```python
from build123d import *

# Parameters (mm, degrees)
F0_W     = 521
F0_H     = 278
F0_W_2   = 117
F0_H_2   = 168
F1_DEPTH = 2


with BuildPart() as f1:
    # F0 (on Front) → F1 (new body)
    with BuildSketch(Plane.XZ):
        Rectangle(F0_W, F0_H)
        with Locations((-147, 0)):
            Rectangle(F0_W_2, F0_H_2, mode=Mode.SUBTRACT)
        Rectangle(F0_W_2, F0_H_2, mode=Mode.SUBTRACT)
        with Locations((147, 0)):
            Rectangle(F0_W_2, F0_H_2, mode=Mode.SUBTRACT)
    extrude(amount=F1_DEPTH)


solid = f1.part
```
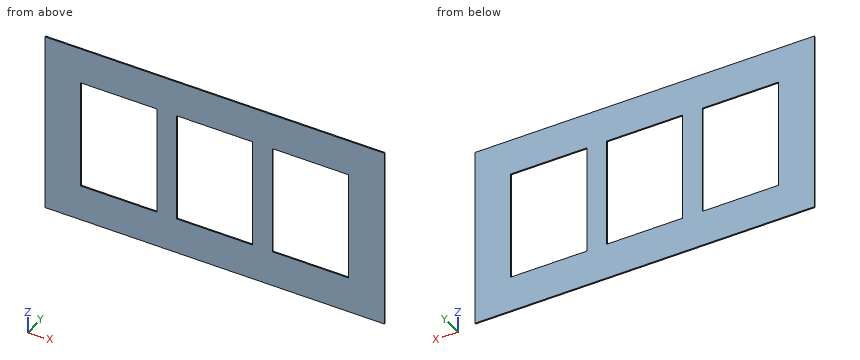
The model under review builds one solid part; all positions refer to its coordinate system, in mm. Round coordinates to 2 decimals unless told otherwise and drop trailing zeros. Order: outer loops, then holes, each group sorted by start corner. A loop starts at its lowest first (then second) coordinate and runs counter-clockwise, first axis right, second up.
Item 1: To check wall thickness, follow probe 1 along X at (y, z) = (-0.2, 8); probe 2 along Z at (x, y) = (168.5, -1.75). State the ranges of each line that lie inside material, in increasing order.
Working result:
probe 1: x = -260.5 to -205.5, -88.5 to -58.5, 58.5 to 88.5, 205.5 to 260.5
probe 2: z = -139 to -84, 84 to 139
Item 2: Add section C-C, the plane y = -0.95. State the section outline as (x, z) points, and give its area (3 significant figures).
Working result:
outline: (-260.5, -139) - (260.5, -139) - (260.5, 139) - (-260.5, 139) - close; hole (-205.5, -84) - (-88.5, -84) - (-88.5, 84) - (-205.5, 84) - close; hole (-58.5, -84) - (58.5, -84) - (58.5, 84) - (-58.5, 84) - close; hole (88.5, -84) - (205.5, -84) - (205.5, 84) - (88.5, 84) - close
area: 85,900 mm2
Item 3: Add section B-B, the plane z = 5. State the section outline as (x, y) points.
Working result:
outline: (-260.5, -2) - (-205.5, -2) - (-205.5, 0) - (-260.5, 0) - close; (-88.5, -2) - (-58.5, -2) - (-58.5, 0) - (-88.5, 0) - close; (58.5, -2) - (88.5, -2) - (88.5, 0) - (58.5, 0) - close; (205.5, -2) - (260.5, -2) - (260.5, 0) - (205.5, 0) - close
Item 4: Add section A-A, the plane x = 149. State the section outline as (y, z) points, and give its area (3 significant figures).
Working result:
outline: (-2, -139) - (0, -139) - (0, -84) - (-2, -84) - close; (-2, 84) - (0, 84) - (0, 139) - (-2, 139) - close
area: 220 mm2
